Check sheet for the drawn part. Datum: minimum x, y, z corner. Units: mm. Coordinates: 2 decimals unless noted, no trailing zeros. Order: outer loops, then holes, each group sorted by start corner. A loop starts at its lowest first (then second) coordinate and runs counter-clockwise, first axis right, second up. Notation, with made-up numbers: (35, 9.25) - (57, 9.25) arc R25 ccw to (57, 36.25) - close; hole circle Ø4 at (25, 76.5). An arc over 180 degrees is marked (long way). Put each result on its own line as item: value.
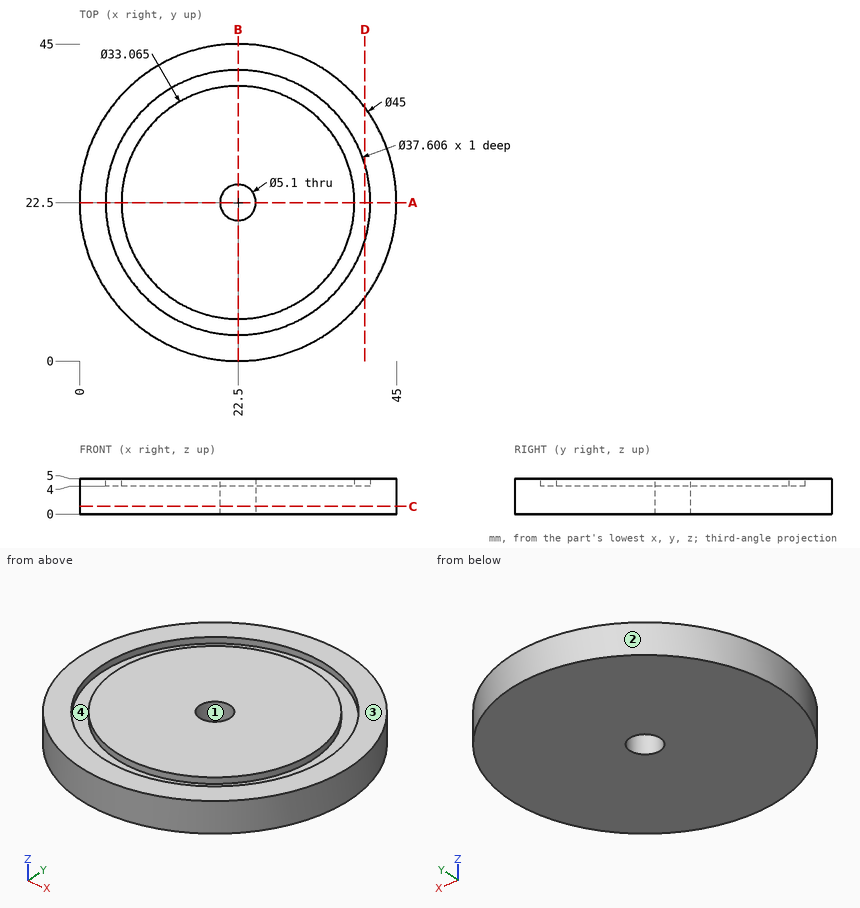
Q1. Section check C-C on z = 1.1. Record the boundary of the cut face in (x, y).
Answer block:
outline: circle Ø45 at (22.5, 22.5); hole circle Ø5.1 at (22.5, 22.5)
Q2. Depth check by flat-ended pin: pin 1 Ø1 at (x, z) = (40.5, 1.5) entering from -Y; pin 2 Ø1 at (y, z) = (16.5, 3) entering from -X; pin 3 Ø1.5 at (x, z) = (34, 4) entering from -Y. Enter the tip coordinate at first touch or a pass-through.
Answer block:
pin 1: stops at y = 8.36
pin 2: stops at x = 0.68
pin 3: stops at y = 2.73
Q3. Thickness scan on L1, parallel to Y at x = 22.5, z = 4.6; L2, parallel to Y at x = 9, z = 4.15 (1 decimal); L3, parallel to X at y = 17.5, z = 4.7. Record the ranges inside material, lowest first. Write a range as [from, to].
Answer block:
L1: y = [0, 3.7], [5.97, 19.95], [25.05, 39.03], [41.3, 45]
L2: y = [4.5, 9.4], [13, 32], [35.6, 40.5]
L3: x = [0.56, 4.37], [6.74, 38.26], [40.63, 44.44]
Q4. Section check D-D on x = 40.5. Record the boundary of the cut face in (y, z), then the cut area to 3 significant figures.
Answer block:
outline: (9, 0) - (36, 0) - (36, 5) - (27.94, 5) - (27.94, 4) - (17.06, 4) - (17.06, 5) - (9, 5) - close
area: 124 mm^2
Q5. Draft check along X on the marked faces 1, 2, 3 and 4. Enter one of: pulls with the +X half, pulls with the -X half, needs draft (parallel to the pull), parting line crosses it, or undercut.
Answer block:
face 1: undercut
face 2: parting line crosses it
face 3: needs draft
face 4: undercut
Q6. Section check A-A on y = 22.5. Record the boundary of the cut face in (x, z), then the cut area to 3 significant figures.
Answer block:
outline: (0, 0) - (19.95, 0) - (19.95, 5) - (5.97, 5) - (5.97, 4) - (3.7, 4) - (3.7, 5) - (0, 5) - close; (25.05, 0) - (45, 0) - (45, 5) - (41.3, 5) - (41.3, 4) - (39.03, 4) - (39.03, 5) - (25.05, 5) - close
area: 195 mm^2
